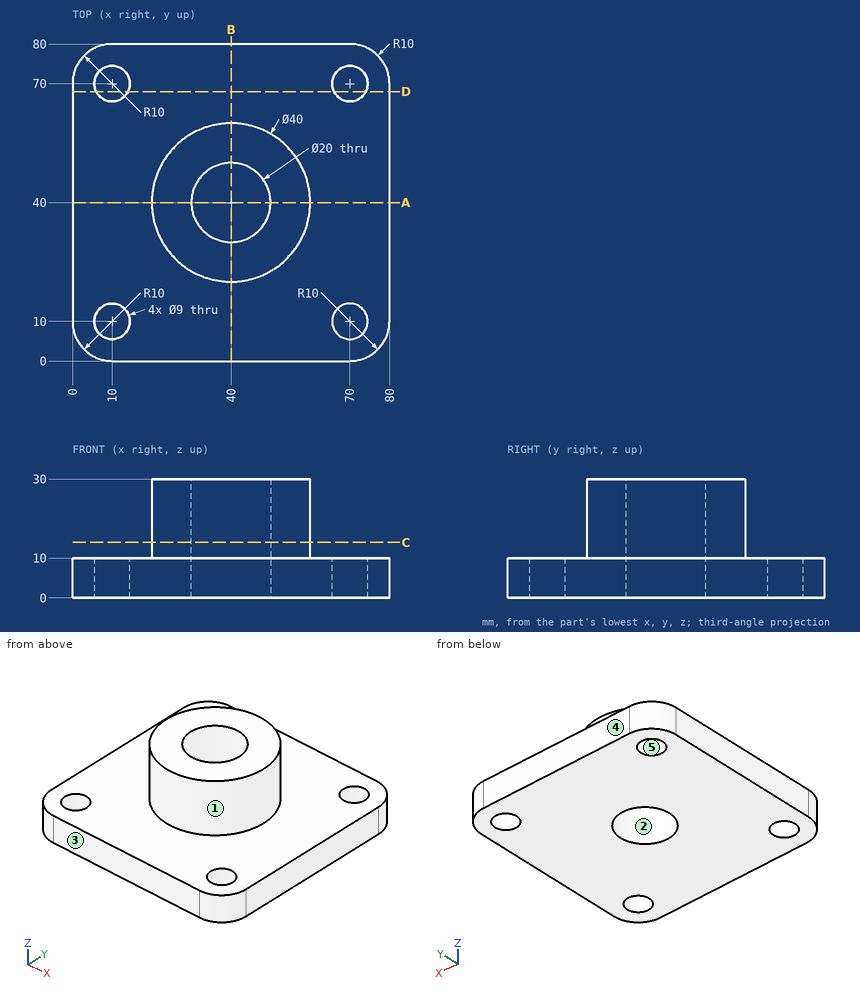
Can you work these out from the drawing? Everything is in mm from the part's minimum corner. A direction names the side the tool comes from. Coordinates: 2 decimals unless noted, no trailing zeros. Loops run counter-clockwise (first coordinate to the right, second up) from the corner with the lowest first, then second, coordinate; pieces in that order, holes last.
1) Which directions (+Z, -Z, +X, -X, +Y, -Y) give clear straight access to the entire face, cutting with the end or side of a thin tool? Please do the marked faces 1 and 2.
2) Imagine slicing it at C-C on z = 14. List the corners of the cut face in (x, y) for me, plus the area to 3 significant figures.
3) For pin 1 (6 mm diameter, centred on y = 57, z = 21.5, fed in from +X); pin 2 (2 mm diameter, centred on x = 59.5, z = 20, fed in from +Y); pin 3 (10 mm diameter, centred on x = 50, z = 16, fed in from +Y), each with a flat end and sliding along its axis, tell me the tip position at first contact or that it passes through.
4) Imagine slicing it at A-A on y = 40. List the corners of the cut face in (x, z) for me, plus the area to 3 significant figures.
5) Thinking about a two-plate mould opening in Y: for the marked faces 3, 4 and 5, which applies, pulls with the +Y half, pulls with the -Y half, needs draft (parallel to the pull), parting line crosses it, or undercut?
6) I need wall thicknesses on probe 1 along X at (y, z) = (70, 2.5); probe 2 along Z at (x, y) = (55, 12). Which ranges of each line are inside material? Lowest first, please.
7) Imagine slicing it at D-D on y = 68. List the corners of the cut face in (x, z) for me, plus the area to 3 significant figures.
Completed:
1. face 1: +Z
1. face 2: +Z, -Z
2. outline: circle Ø40 at (40, 40); hole circle Ø20 at (40, 40)
2. area: 942 mm2
3. pin 1: stops at x = 54.28
3. pin 2: stops at y = 47.6
3. pin 3: stops at y = 59.36
4. outline: (0, 0) - (30, 0) - (30, 30) - (20, 30) - (20, 10) - (0, 10) - close; (50, 0) - (80, 0) - (80, 10) - (60, 10) - (60, 30) - (50, 30) - close
4. area: 1,000 mm2
5. face 3: pulls with the -Y half
5. face 4: pulls with the +Y half
5. face 5: undercut
6. probe 1: x = 0 to 5.5, 14.5 to 65.5, 74.5 to 80
6. probe 2: z = 0 to 10
7. outline: (0, 0) - (5.97, 0) - (5.97, 10) - (0, 10) - close; (14.03, 0) - (65.97, 0) - (65.97, 10) - (14.03, 10) - close; (74.03, 0) - (80, 0) - (80, 10) - (74.03, 10) - close
7. area: 639 mm2
